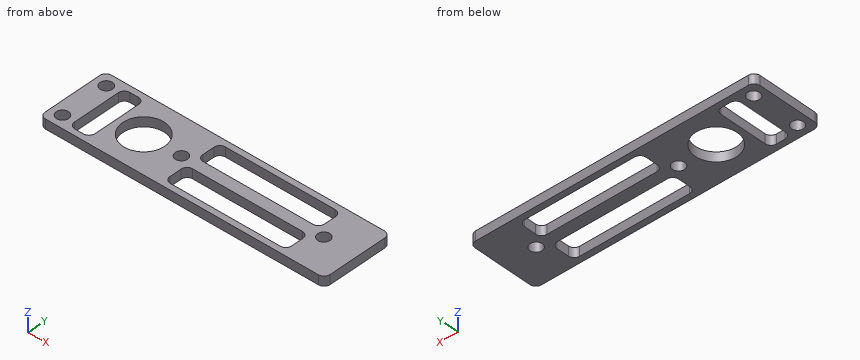
from build123d import *

# Parameters (mm, degrees)
SKETCH1_W           = 96
SKETCH1_H           = 24
SKETCH1_R           = 7.05
SKETCH1_R_2         = 2.05
SKETCH1_W_2         = 41
SKETCH1_H_2         = 8.061482978
SKETCH1_W_3         = 6.9
SKETCH1_H_3         = 20
BOSS_EXTRUDE1_DEPTH = 3.175
FILLET1_R           = 2


with BuildPart() as part:
    # Sketch1 → Boss-Extrude1 (new body)
    with BuildSketch(Plane.XY):
        Rectangle(SKETCH1_W, SKETCH1_H)
        with Locations((-24, 0)):
            Circle(SKETCH1_R, mode=Mode.SUBTRACT)
        with Locations((-11.31, 0)):
            Circle(SKETCH1_R_2, mode=Mode.SUBTRACT)
        with Locations((36.69, 0)):
            Circle(SKETCH1_R_2, mode=Mode.SUBTRACT)
        with Locations((-44, 8)):
            Circle(SKETCH1_R_2, mode=Mode.SUBTRACT)
        with Locations(Location((-44, -8, 0), (0, 0, 180))):
            Circle(SKETCH1_R_2, mode=Mode.SUBTRACT)
        with Locations((12.745931911, -5.969258511)):
            Rectangle(SKETCH1_W_2, SKETCH1_H_2, mode=Mode.SUBTRACT)
        with Locations((12.745931911, 5.969258511)):
            Rectangle(SKETCH1_W_2, SKETCH1_H_2, mode=Mode.SUBTRACT)
        with Locations((-36.5, 0)):
            Rectangle(SKETCH1_W_3, SKETCH1_H_3, mode=Mode.SUBTRACT)
    extrude(amount=BOSS_EXTRUDE1_DEPTH)

    # Fillet1
    fillet1_edges = [part.edges().sort_by_distance(p)[0] for p in [
        (-7.754068089, 10, 1.5875),
        (-7.754068089, 1.938517022, 1.5875),
        (33.245931911, 1.938517022, 1.5875),
        (33.245931911, 10, 1.5875),
        (-7.754068089, -1.938517022, 1.5875),
        (-7.754068089, -10, 1.5875),
        (33.245931911, -10, 1.5875),
        (33.245931911, -1.938517022, 1.5875),
        (-39.95, 10, 1.5875),
        (-39.95, -10, 1.5875),
        (-33.05, -10, 1.5875),
        (-33.05, 10, 1.5875),
        (-48, 12, 1.5875),
        (48, 12, 1.5875),
        (48, -12, 1.5875),
        (-48, -12, 1.5875),
    ]]
    fillet(fillet1_edges, radius=FILLET1_R)


solid = part.part
The model under review builds one solid part; all positions refer to its coordinate system, in mm. Round coordinates to 2 decimals unless told otherwise and drop trailing zeros. Order: outer loops, then holes, each group sorted by start corner. A loop starts at its lowest first (then second) coordinate and runs counter-clockwise, first axis right, second up. Notation, with made-up numbers: (-29.75, 41.25) -> (-2.75, 41.25) arc R36 cw to (-2.75, 77.25) -> close; hole circle Ø9 at (62.5, -11). An arc over 180 degrees is marked (long way). Return JSON: item names as keys, results as strings.
1. Take a section at D-D (x = -11.31). Write out the cut boundary in (y, z) (3 decimals).
Answer block:
{"outline": "(-12, 0) -> (-2.05, 0) -> (-2.05, 3.175) -> (-12, 3.175) -> close; (2.05, 0) -> (12, 0) -> (12, 3.175) -> (2.05, 3.175) -> close"}
2. For L1, parallel to X at y = -8, z = 1.65; L2, parallel to Y at x = 8, z = 0.7; L3, parallel to Y at x = -6, z = 0.7, list the stretches that pass through material, from the lowest coordinate up. Write a range as [from, to].
Answer block:
{"L1": "x = [-48, -46.05], [-41.95, -39.95], [-33.05, -7.75], [33.25, 48]", "L2": "y = [-12, -10], [-1.94, 1.94], [10, 12]", "L3": "y = [-12, -9.98], [-1.95, 1.95], [9.98, 12]"}
3. Insertion check: P1, Ø3, axis at x = -34, y = -2, coming from the -Z side. The pin has a flat end and moves straight along its axis. Give the tip position at first contact, or say it passes through.
Answer block:
{"P1": "stops at z = 0"}
4. Take a section at C-C (y = 0). Write out the cut boundary in (x, z) (3 decimals).
Answer block:
{"outline": "(-48, 0) -> (-39.95, 0) -> (-39.95, 3.175) -> (-48, 3.175) -> close; (-33.05, 0) -> (-31.05, 0) -> (-31.05, 3.175) -> (-33.05, 3.175) -> close; (-16.95, 0) -> (-13.36, 0) -> (-13.36, 3.175) -> (-16.95, 3.175) -> close; (-9.26, 0) -> (34.64, 0) -> (34.64, 3.175) -> (-9.26, 3.175) -> close; (38.74, 0) -> (48, 0) -> (48, 3.175) -> (38.74, 3.175) -> close"}
5. Take a section at B-B (x = -44). Write out the cut boundary in (y, z) (3 decimals), then the cut area to 3 significant figures.
Answer block:
{"outline": "(-12, 0) -> (-10.05, 0) -> (-10.05, 3.175) -> (-12, 3.175) -> close; (-5.95, 0) -> (5.95, 0) -> (5.95, 3.175) -> (-5.95, 3.175) -> close; (10.05, 0) -> (12, 0) -> (12, 3.175) -> (10.05, 3.175) -> close", "area": "50.2 mm²"}
6. Take a section at A-A (x = -24). Write out the cut boundary in (y, z) (3 decimals), then the cut area to 3 significant figures.
Answer block:
{"outline": "(-12, 0) -> (-7.05, 0) -> (-7.05, 3.175) -> (-12, 3.175) -> close; (7.05, 0) -> (12, 0) -> (12, 3.175) -> (7.05, 3.175) -> close", "area": "31.4 mm²"}
